```python
from build123d import *

# Parameters (mm, degrees)
SKETCH1_R           = 31.75
BOSS_EXTRUDE1_DEPTH = 155.575
SKETCH2_R           = 25.4
BOSS_EXTRUDE2_DEPTH = 76.2
BOSS_EXTRUDE3_START = 76.2
SKETCH3_R           = 25.4
BOSS_EXTRUDE3_DEPTH = 76.2
SKETCH18_R          = 17.4625
BOSS_EXTRUDE6_DEPTH = 57.15
SKETCH20_W          = 7.9248
SKETCH20_H          = 7.9248
CUT_EXTRUDE1_DEPTH  = 44.45


with BuildPart() as part:
    # Sketch1 → Boss-Extrude1 (new, symmetric)
    with BuildSketch(Plane.XY):
        Circle(SKETCH1_R)
    extrude(amount=BOSS_EXTRUDE1_DEPTH, both=True)

    # Sketch2 → Boss-Extrude2 (add)
    with BuildSketch(Plane.XY.offset(155.575)):
        with Locations(Location((0, 0, 0), (0, 0, 180))):
            Circle(SKETCH2_R)
    extrude(amount=BOSS_EXTRUDE2_DEPTH)

    # Sketch3 → Boss-Extrude3 (add)
    with BuildSketch(Plane(origin=(0, 0, -155.575), x_dir=(-1, 0, 0), z_dir=(0, 0, -1)).offset(BOSS_EXTRUDE3_START)):
        Circle(SKETCH3_R)
    extrude(amount=-BOSS_EXTRUDE3_DEPTH)

    # Sketch18 → Boss-Extrude6 (add)
    with BuildSketch(Plane.XY.offset(231.775)):
        Circle(SKETCH18_R)
    extrude(amount=BOSS_EXTRUDE6_DEPTH)

    # Sketch20 → Cut-Extrude1 (cut)
    with BuildSketch(Plane.XY.offset(288.925)):
        with Locations((0, 17.4625)):
            Rectangle(SKETCH20_W, SKETCH20_H)
    extrude(amount=-CUT_EXTRUDE1_DEPTH, mode=Mode.SUBTRACT)


solid = part.part
```
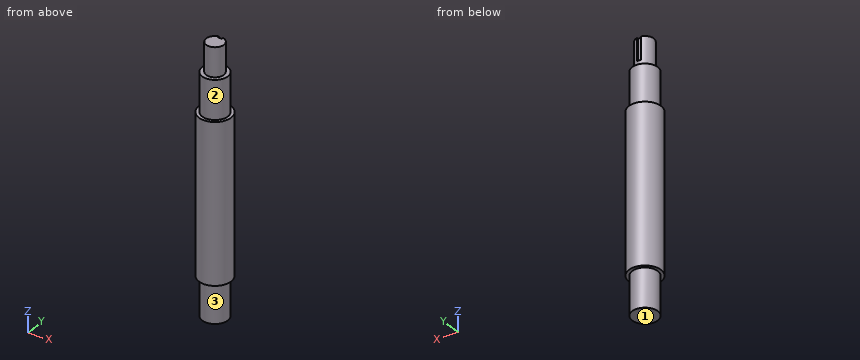
Can you work these out from the model? Positions are in its coordinate system, mm. Face numbers are marked on the shaded views. A direction names the side the tool comes from. Give positions to 0.01 mm unless a question says otherwise; leave off trailing zeros. Loops run counter-clockwise (first coordinate to the right, second up) from the corner with the lowest first, then second, coordinate; pieces in that order, holes last. Notation, with made-up numbers: M -33.5,-38 L -26.5,-38 A24 ccw -26.5,-20 Z; hole C -16,72 d4. An arc over 180 degrees is marked long. Use CSV: the item, a comma, the result in double quotes. Start each with the question number.
1. Imagine slicing it at B-B, the plane x = -11. Write out the boundary of the cut face in (y, z) (3 decimals), plus the area to 3 significant figures.
2. For P1, Ø2, axis at x = -2, y = 15, coming from the +Z side (3 decimals); P2, Ø2, axis at y = -6.5, z = -143, coming from the -X side; P3, Ø3, axis at x = -13.5, z = 18.5, coming from the -Y side, each with a flat end and sliding along its axis, tell me the tip position at first contact or that it passes through.
3. On a 3-axis mill with a long thin cutter (end or side, diameter ignored), from which of +Z, -Z, +X, -X, +Y, -Y can I reach the whole of each face in a straight line? I mean the marked faces 1, 2 and 3. Say none if no direction works.
4. Imagine slicing it at C-C, the plane z = -30.5. Write out the boundary of the cut face in (x, y), plus the area to 3 significant figures.
5. If I drill on L1, parallel to Z at x = 21, y = -9 (3 decimals); L2, parallel to X at y = 1.5, z = 88; L3, parallel to Z at x = -26.5, y = 13.5 (3 decimals), over which ranges is the centre line in solid material (lowest first)?
Response values:
1,outline,"M -29.784,-155.575 L -22.895,-155.575 L -22.895,-231.775 L 22.895,-231.775 L 22.895,-155.575 L 29.784,-155.575 L 29.784,155.575 L 22.895,155.575 L 22.895,231.775 L 13.562,231.775 L 13.562,288.925 L -13.562,288.925 L -13.562,231.775 L -22.895,231.775 L -22.895,155.575 L -29.784,155.575 Z"
1,area,"27,100 mm^2"
2,P1,"z = 244.475"
2,P2,"x = -31.27"
2,P3,"y = -29.39"
3,face 1,"-Z, +X, -X, +Y, -Y"
3,face 2,"+Z"
3,face 3,"-Z"
4,outline,"C 0,0 d63.5"
4,area,"3,170 mm^2"
5,L1,"-231.775 to 231.775"
5,L2,"-31.71 to 31.71"
5,L3,"-155.575 to 155.575"
